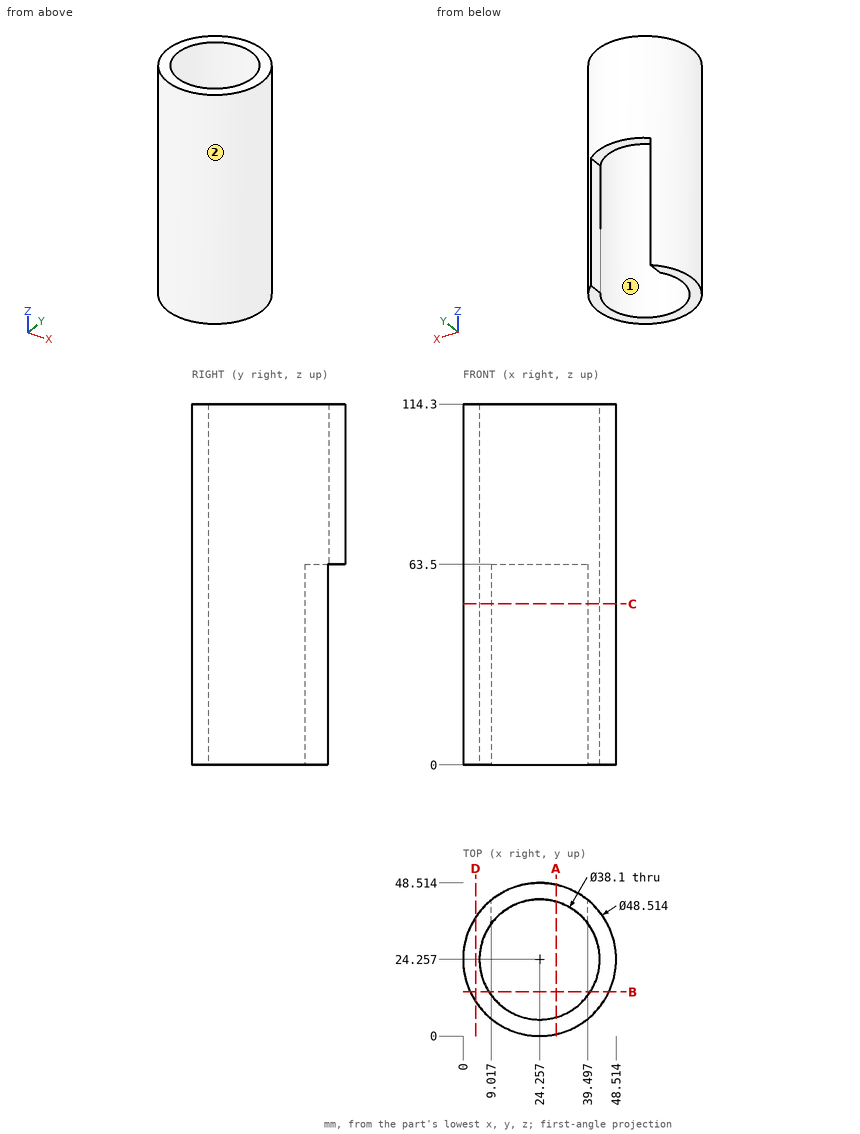
The figure shows three views and two pictorial views of one solid part (mm, origin at its lowest corner). Answer the questions. Round coordinates to 2 decimals unless told otherwise and drop trailing zeros. Write each loop counter-clockwise with the first axis right and the second up, starting at its lowest first coordinate (ties: lowest second). Pieces come first, ordered by that corner, then holes. Notation, with made-up numbers: (10.5, -33) - (43.5, -33) arc R30 cw to (43.5, -7) - close; hole circle Ø10 at (-35.75, 1). An arc over 180 degrees is marked (long way). Answer in a Markdown table with one row per item. Add a question column.
1. A cutting plane is placed at B-B, the plane y = 14. Determine the outline of the cut face in (x, z).
2. Given pin 1 (2 mm diameter, centred on x = 5.5, z = 22.5, fed in from +Y); pin 2 (3 mm diameter, centred on x = 31.5, z = 85, fed in from +Y); pin 3 (12 mm diameter, centred on x = 34.5, z = 85, fed in from -Y); pin 4 (10 mm diameter, centred on x = 24, y = 13, fed in from -Z), each flat-ended and moving along its own axis, determine where each tip first touches the part or whether it passes through.
3. A cutting plane is placed at D-D, the plane x = 4. Determine the outline of the cut face in (y, z), and give its area (3 significant figures).
4. Find the intervals of material crossed by line 1 along X through (y, z) = (25, 88); line 2 along X through (y, z) = (19.5, 64); line 3 along Y through (x, z) = (23, 72), in increasing order. Write a range as from..to.
5. The mould has two halves that part along X. Classify the marked faces 1 and 2: +X half, -X half, draft (parallel to the pull), parting line (faces both ways), or undercut.
6. A cutting plane is placed at C-C, the plane z = 51. Determine the outline of the cut face in (x, y).
7. A cutting plane is placed at A-A, the plane x = 29.5. Determine the outline of the cut face in (y, z).
Worked out:
| question | item | result |
|---|---|---|
| 1 | outline | (2.28, 0) - (8.2, 0) - (8.2, 114.3) - (2.28, 114.3) - close; (40.31, 0) - (46.24, 0) - (46.24, 114.3) - (40.31, 114.3) - close |
| 2 | pin 1 | y = 40.78 |
| 2 | pin 2 | y = 47.82 |
| 2 | pin 3 | y = 0.37 |
| 2 | pin 4 | through |
| 3 | outline | (10.91, 0) - (37.6, 0) - (37.6, 114.3) - (10.91, 114.3) - close |
| 3 | area | 3,050 mm^2 |
| 4 | line 1 | 0.01..5.22, 43.29..48.5 |
| 4 | line 2 | 0.47..5.81, 42.7..48.04 |
| 4 | line 3 | 0.03..5.25, 43.27..48.48 |
| 5 | face 1 | undercut |
| 5 | face 2 | parting line |
| 6 | outline | (9.02, 35.69) - (9.02, 43.13) arc R24.26 ccw (long way) to (39.5, 43.13) - (39.5, 35.69) arc R19.05 cw (long way) to start |
| 7 | outline | (0.57, 0) - (5.94, 0) - (5.94, 114.3) - (0.57, 114.3) - close; (42.57, 63.5) - (47.94, 63.5) - (47.94, 114.3) - (42.57, 114.3) - close |
